Source: three-view drawing plus pictorial views. Frame: mm from the lowest corner of the part. A direction names the side the tool comes from. Round coordinates to 2 decimals unless told otherwise and drop trailing zeros. Loops run counter-clockwise (first coordinate to the right, second up) from the corner with the lowest first, then second, coordinate; pieces in that order, holes last. Notation, with made-up numbers: M 21.25,63 L 25.25,63 A19 ccw 25.25,86 Z; hole C 45,-24.75 d5. An arc over 180 degrees is marked long. Answer as a JSON object with one key per item and string values.
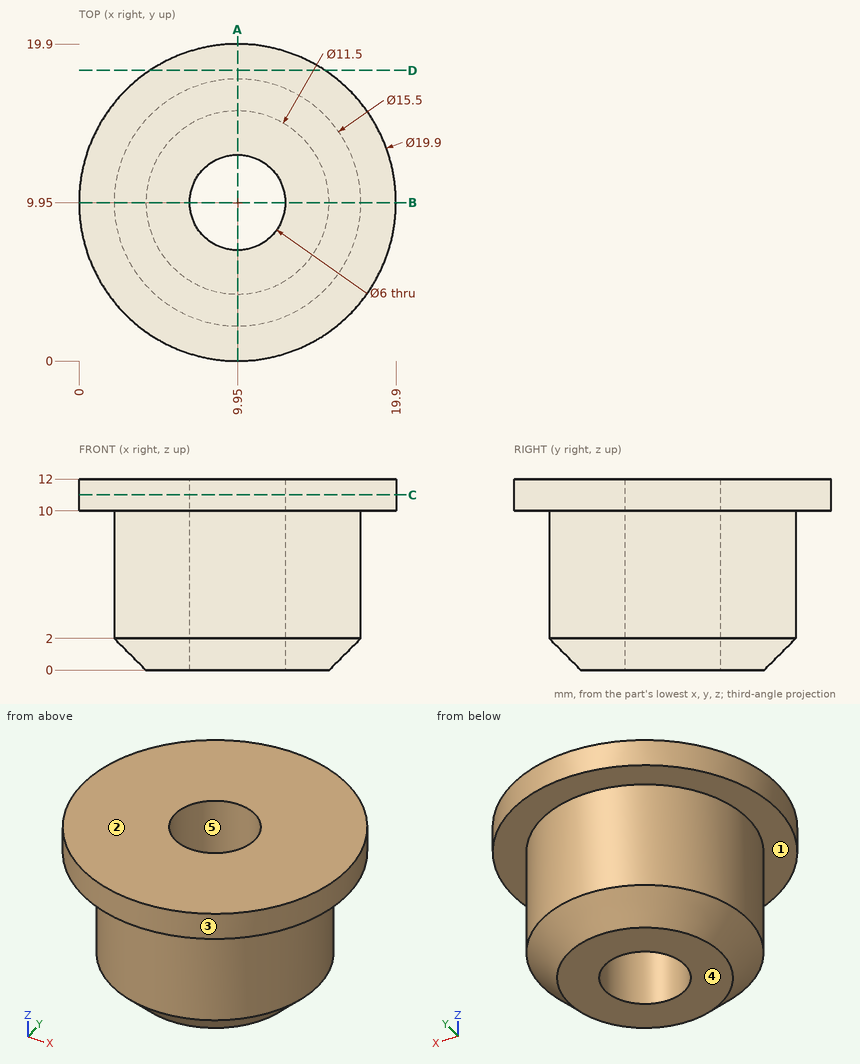
1) Cut plane D-D on y = 18.25. Return the cut outline in (x, z), and give its area (4 significant figures).
Geometry results:
{"outline": "M 4.46,10 L 15.44,10 L 15.44,12 L 4.46,12 Z", "area": "21.95 mm2"}
2) Pull-direction query (Y, two-part tool) for the marked faces 3, 4 and 5; classes: +Y half, -Y half, draft (parallel to the pull), parting line (faces both ways), or undercut.
Geometry results:
{"face 3": "parting line", "face 4": "draft", "face 5": "undercut"}
3) Cut plane C-C on z = 11. Return the cut outline in (x, y), and give its area (3 significant figures).
Geometry results:
{"outline": "C 9.95,9.95 d19.9; hole C 9.95,9.95 d6", "area": "283 mm2"}
4) Line query: probe 1 along Y at (x, z) = (9.95, 8.5); probe 2 along Z at (x, y) = (4.5, 16.5); probe 3 along Y at (x, z) = (12, 4.75). Output: solid intervals per line, ascending.
Geometry results:
{"probe 1": "2.2 to 6.95, 12.95 to 17.7", "probe 2": "10 to 12", "probe 3": "2.48 to 7.76, 12.14 to 17.42"}
5) First-contact query: pin 1 (1.5 mm diameter, centred on x = 5.5, z = 1.5, fed in from -Y); pin 2 (1 mm diameter, centred on y = 7.5, z = 10.5, fed in from -X). Flat tips, straight axial feed; report the tip coordinate or a pass-through.
Geometry results:
{"pin 1": "y = 3.25", "pin 2": "x = 0.19"}
6) Set-up query: the marked faces 1 and 2. Return all of +Z, -Z, +X, -X, +Y, -Y with unobstructed straight access to the full face (end or side cutting, diameter ignored); none if empty.
Geometry results:
{"face 1": "-Z", "face 2": "+Z, +X, -X, +Y, -Y"}
7) Cut plane A-A on x = 9.95. Return the cut outline in (y, z), and give its area (3 significant figures).
Geometry results:
{"outline": "M 0,10 L 2.2,10 L 2.2,2 L 4.2,0 L 6.95,0 L 6.95,12 L 0,12 Z; M 12.95,0 L 15.7,0 L 17.7,2 L 17.7,10 L 19.9,10 L 19.9,12 L 12.95,12 Z", "area": "119 mm2"}
